```python
from build123d import *

# Parameters (mm, degrees)
F0_W           = 32
F0_H           = 77
F0_R           = 2
F1_DEPTH       = 6
F2_R           = 2
F4_D           = 4
F4_DEPTH       = 10
F4_CSINK_D     = 8
F4_CSINK_ANGLE = 90


with BuildPart() as f1:
    # F0 (on Top) → F1 (new body)
    with BuildSketch(Plane.XY):
        Rectangle(F0_W, F0_H)
        with Locations((-6, -26.5)):
            Circle(F0_R, mode=Mode.SUBTRACT)
        with Locations((-6, 13.5)):
            Circle(F0_R, mode=Mode.SUBTRACT)
    extrude(amount=F1_DEPTH)

    # F2
    f2_edges = [f1.edges().sort_by_distance(p)[0] for p in [
        (-16, 38.5, 3),
        (16, 38.5, 3),
        (16, -38.5, 3),
        (-16, -38.5, 3),
    ]]
    fillet(f2_edges, radius=F2_R)

    # F4
    with Locations(Plane.XY.offset(6)):
        with Locations((-6, 13.5), (-6, -26.5)):
            CounterSinkHole(F4_D / 2, F4_CSINK_D / 2, depth=F4_DEPTH, counter_sink_angle=F4_CSINK_ANGLE)


solid = f1.part
```
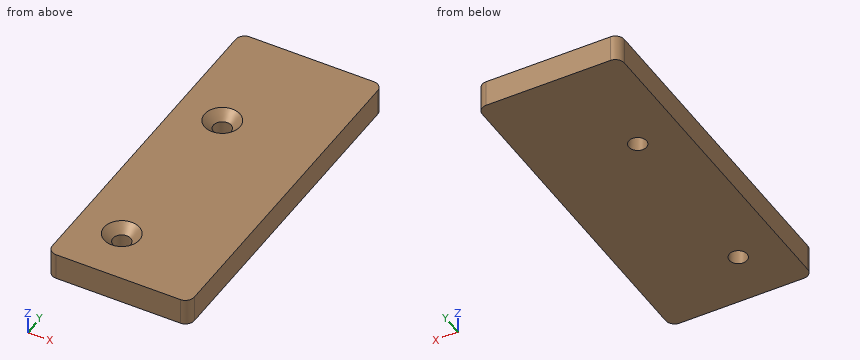
Part model, mm, in its own coordinate system. Round coordinates to 2 decimals unless told otherwise and drop trailing zeros. Loops run counter-clockwise (first coordinate to the right, second up) from the corner with the lowest first, then second, coordinate; pieces in that order, holes last.
Item 1: Cut at B-B, the plane x = -6. Give the cut face in (y, z), then the cut area to 3 significant figures.
Item 2: Cut at C-C, the plane z = 4.75. Give the cut face in (x, y), then the cut area to 3 significant figures.
Item 3: Cut at A-A, the plane y = 13.5. Give the cut face in (x, z), then the cut area to 3 significant figures.
Item 4: Drop a flat-ended pin along its axis: P1, Ø2.5, axis at x = -6, y = -26.5, coming from the -Z side. Give the stop position or say it passes through.
Item 5: Drill centre lines: line 1 (Y direction, x = -6, z = 1.1); line 2 (X direction, y = 13.5, z = 2.85); line 3 (Y direction, x = -7, z = 5.75). Where is each one in solid material? Low to high.
A:
1. outline: (-38.5, 0) - (-28.5, 0) - (-28.5, 4) - (-30.5, 6) - (-38.5, 6) - close; (-24.5, 0) - (11.5, 0) - (11.5, 4) - (9.5, 6) - (-22.5, 6) - (-24.5, 4) - close; (15.5, 0) - (38.5, 0) - (38.5, 6) - (17.5, 6) - (15.5, 4) - close
1. area: 406 mm2
2. outline: (-16, -36.5) arc R2 ccw to (-14, -38.5) - (14, -38.5) arc R2 ccw to (16, -36.5) - (16, 36.5) arc R2 ccw to (14, 38.5) - (-14, 38.5) arc R2 ccw to (-16, 36.5) - close; hole circle Ø5.5 at (-6, -26.5); hole circle Ø5.5 at (-6, 13.5)
2. area: 2,410 mm2
3. outline: (-16, 0) - (-8, 0) - (-8, 4) - (-10, 6) - (-16, 6) - close; (-4, 0) - (16, 0) - (16, 6) - (-2, 6) - (-4, 4) - close
3. area: 164 mm2
4. P1: passes through
5. line 1: y = -38.5 to -28.5, -24.5 to 11.5, 15.5 to 38.5
5. line 2: x = -16 to -8, -4 to 16
5. line 3: y = -38.5 to -30.11, -22.89 to 9.89, 17.11 to 38.5
